from build123d import *

# Parameters (mm, degrees)
BOSS_EXTRUDE2_DEPTH = 22
SKETCH3_W           = 4
SKETCH3_H           = 16
BOSS_EXTRUDE3_DEPTH = 1
SKETCH6_W           = 5
SKETCH6_H           = 1
BOSS_EXTRUDE4_DEPTH = 22
CUT_EXTRUDE1_REACH  = 38.851
SKETCH7_W           = 21
SKETCH7_H           = 3.4


with BuildPart() as part:
    # Sketch2 → Boss-Extrude2 (new body)
    with BuildSketch(Plane.XY):
        Polygon((11.2, -6.9), (11.2, 11.1), (-11.2, 11.1), (-11.2, -5.9), (-15.2, -5.9), (-15.2, 10.1), (-16.2, 10.1), (-16.2, -6.9), (-10.2, -6.9), (-10.2, 10.1), (10.2, 10.1), (10.2, -6.9), align=None)
    extrude(amount=BOSS_EXTRUDE2_DEPTH)

    # Sketch3 → Boss-Extrude3 (add)
    with BuildSketch(Plane(origin=(0, 0, 0), x_dir=(-1, 0, 0), z_dir=(0, 0, -1))):
        with Locations((13.2, 2.1)):
            Rectangle(SKETCH3_W, SKETCH3_H)
    extrude(amount=-BOSS_EXTRUDE3_DEPTH)

    # Sketch6 → Boss-Extrude4 (add)
    with BuildSketch(Plane.XY.offset(22)):
        with Locations((-13.7, 10.6)):
            Rectangle(SKETCH6_W, SKETCH6_H)
    extrude(amount=-BOSS_EXTRUDE4_DEPTH)

    # Sketch7 → Cut-Extrude1 (cut, up to next)
    with BuildSketch(Plane.ZY.offset(16.2), mode=Mode.PRIVATE) as cut_extrude1_sk1:
        with Locations((11.5, -4.2)):
            Rectangle(SKETCH7_W, SKETCH7_H)
    cut_extrude1_tool1 = extrude(cut_extrude1_sk1.sketch, amount=-CUT_EXTRUDE1_REACH, mode=Mode.PRIVATE) & part.part
    # Sketch7 → Cut-Extrude1 (cut, up to next)
    with BuildSketch(Plane.ZY.offset(16.2), mode=Mode.PRIVATE) as cut_extrude1_sk2:
        with Locations((11.5, 8.4)):
            Rectangle(SKETCH7_W, SKETCH7_H)
    cut_extrude1_tool2 = extrude(cut_extrude1_sk2.sketch, amount=-CUT_EXTRUDE1_REACH, mode=Mode.PRIVATE) & part.part
    add(cut_extrude1_tool1.solids().sort_by_distance((-16.2, -4.2, 11.5))[0], mode=Mode.SUBTRACT)
    add(cut_extrude1_tool2.solids().sort_by_distance((-16.2, 8.4, 11.5))[0], mode=Mode.SUBTRACT)


solid = part.part
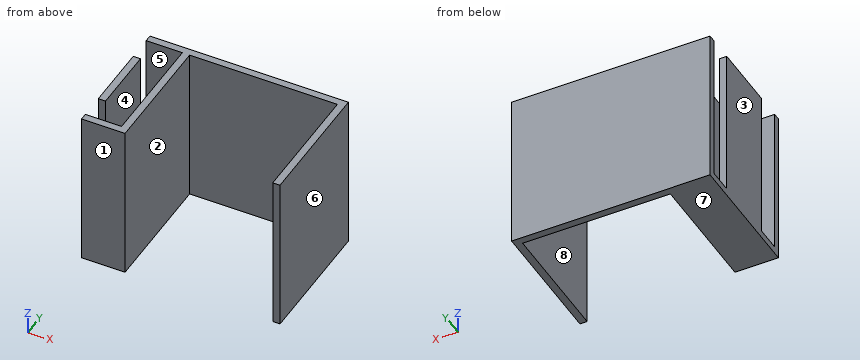
Can you work these out from the model? Positions are in its coordinate system, mm. Face numbers are marked on the shaded views. A direction names the side the tool comes from. Coordinates: 2 decimals unless noted, no trailing zeros. Write each loop counter-clockwise with the first axis right and the second up, starting at its lowest first coordinate (ties: lowest second). Pieces come first, ordered by that corner, then holes. Notation, with made-up numbers: M -3.5,15 L 15.5,15 A4 cw 15.5,22 Z; hole C 15.5,78.25 d1. An arc over 180 degrees is marked long. Use one line per item in the form item = value.
Q1. I need wall thicknesses on line 1 along X through (y, z) = (6.5, 9.75); line 2 along X through (y, z) = (8, 5); line 3 along Y through (x, z) = (-14.75, 19). Which ranges of each line are inside material? Lowest first, please. Write a range as from..to.
Model answer:
line_1 = -16.2..-15.2, -11.2..-10.2, 10.2..11.2
line_2 = -11.2..-10.2, 10.2..11.2
line_3 = -6.9..-5.9, 10.1..11.1
Q2. If we section it at D-D (x = 7): Write out the boundary of the cut face in (y, z), then the cut area to 3 significant figures.
Model answer:
outline = M 10.1,0 L 11.1,0 L 11.1,22 L 10.1,22 Z
area = 22.0 mm^2
Q3. For the marked faces 4, 5, 6, 7 and 8, which set-ups out of +Z, -Z, +X, -X, +Y, -Y let a thin tool reach every point of the face, with its end or its side?
Model answer:
face_4 = +Z
face_5 = +Z, -X
face_6 = +Z, -Z, +X, +Y, -Y
face_7 = -Z, +X, -X, +Y, -Y
face_8 = +Z, -Z, -Y
Q4. We'd pull the mould along X, two halves only. Please class the marked faces 1, 2 and 3: +X half, -X half, draft (parallel to the pull), parting line (faces both ways), or undercut.
Model answer:
face_1 = draft
face_2 = undercut
face_3 = -X half
Q5. If we section it at B-B (z = 7.25): Write out the boundary of the cut face in (x, y), then the cut area to 3 significant figures.
Model answer:
outline = M -16.2,-6.9 L -10.2,-6.9 L -10.2,10.1 L 10.2,10.1 L 10.2,-6.9 L 11.2,-6.9 L 11.2,11.1 L -16.2,11.1 L -16.2,10.1 L -11.2,10.1 L -11.2,-5.9 L -16.2,-5.9 Z; M -16.2,-2.5 L -15.2,-2.5 L -15.2,6.7 L -16.2,6.7 Z
area = 75.6 mm^2
Q6. If we section it at C-C (y = 1.75): Write out the boundary of the cut face in (x, z), then the cut area to 3 significant figures.
Model answer:
outline = M -16.2,0 L -10.2,0 L -10.2,22 L -11.2,22 L -11.2,1 L -15.2,1 L -15.2,22 L -16.2,22 Z; M 10.2,0 L 11.2,0 L 11.2,22 L 10.2,22 Z
area = 70.0 mm^2
Q7. For P1, Ø2, axis at x = 7.5, y = -1.5, coming from the -Z side; P2, Ø6, axis at x = -3, z = 7.5, coming from the -Y side; P3, Ø5.5, axis at x = -14.5, y = 0, coming from the +Z side, each with a flat end and sliding along its axis, tell me the tip position at first contact or that it passes through.
Model answer:
P1 = through
P2 = 10.1
P3 = 22
Q8. If we section it at A-A (y = -5.25): Write out the boundary of the cut face in (x, z).
Model answer:
outline = M -16.2,0 L -10.2,0 L -10.2,22 L -11.2,22 L -11.2,1 L -16.2,1 Z; M 10.2,0 L 11.2,0 L 11.2,22 L 10.2,22 Z
